Answer from the drawing. Dimensions are ordinates in mm from the lowest x, y and z of the part. A direction names the side the tool comes from. Give positions to 0.01 mm unless a question says otherwise; leave off trailing zeros. Order: outer loops, then holes, each group sorted by start corner. A loop starts at its lowest first (then second) coordinate and runs counter-clockwise, first axis right, second up.
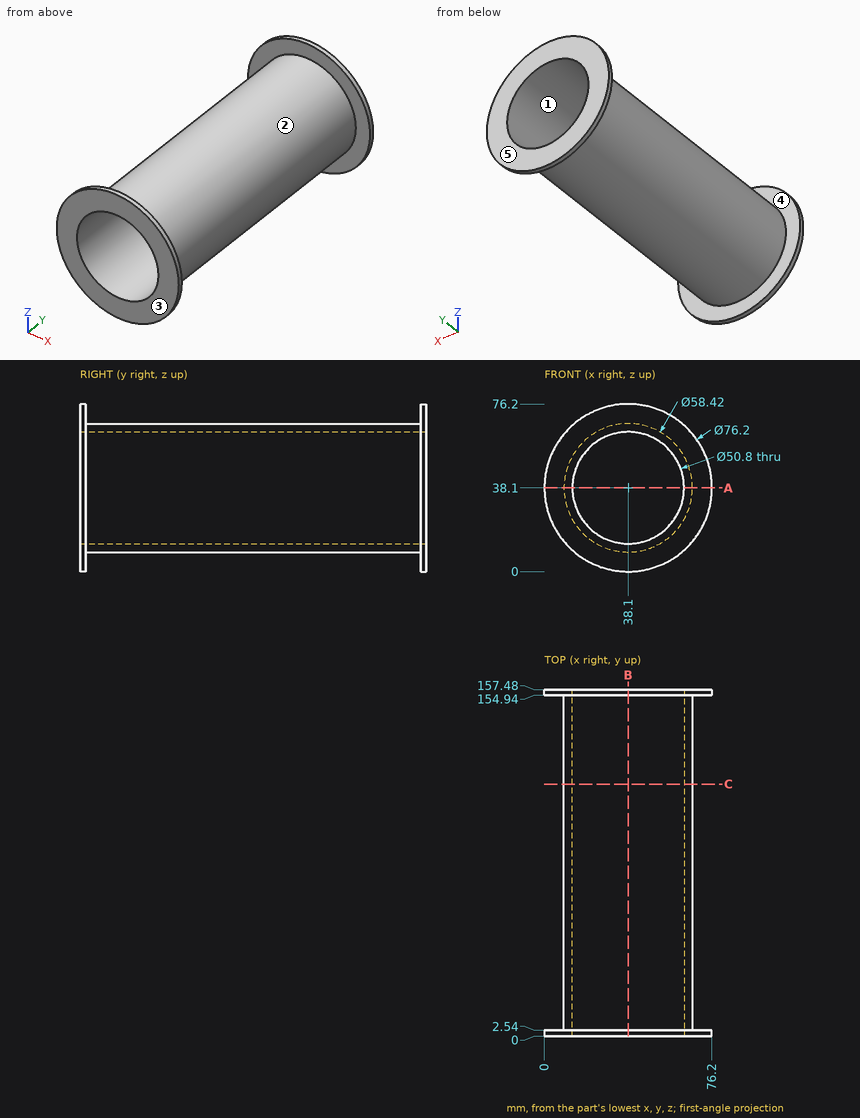
1. Which of the six approach directions +Z, -Z, +X, -X, +Y, -Y give full straight-line access (tool end or side, diameter ignored) to the marked faces 4 and 5?
Findings below:
face 4: none
face 5: +Z, -Z, +X, -X, +Y
2. The part is cut by section C-C (y = 114.5). Write down the section's boundary in (x, z).
Findings below:
outline: circle Ø58.42 at (38.1, 38.1); hole circle Ø50.8 at (38.1, 38.1)
3. The mould has two halves that part along Z. Classify the marked faces 1, 2 and 3: pulls with the +Z half, pulls with the -Z half, needs draft (parallel to the pull), parting line crosses it, or undercut.
Findings below:
face 1: undercut
face 2: parting line crosses it
face 3: needs draft
4. Given P1, Ø8, axis at y = 80.5, z = 66, coming from the +X side; P2, Ø1.5, axis at x = 21, y = 104.5, coming from the -Z side; P3, Ø6, axis at y = 120.5, z = 56, coming from the -X side; P4, Ø3, axis at x = 36.5, z = 16, coming from the -Y side, each flat-ended and moving along its own axis, determine where each tip first touches the part or whether it passes through.
Findings below:
P1: stops at x = 54.89
P2: stops at z = 13.89
P3: stops at x = 12.98
P4: passes through
5. Straight lines are drawn through the part: probe 1 along X at (y, z) = (89, 38); probe 2 along Y at (x, z) = (29.5, 5). For each, find the intervals that lie inside material, in ascending order.
Findings below:
probe 1: x = 8.89 to 12.7, 63.5 to 67.31
probe 2: y = 0 to 2.54, 154.94 to 157.48
6. The part is cut by section B-B (x = 38.1). Write down the section's boundary in (y, z), then the cut area to 3 significant figures.
Findings below:
outline: (0, 0) - (2.54, 0) - (2.54, 8.89) - (154.94, 8.89) - (154.94, 0) - (157.48, 0) - (157.48, 12.7) - (0, 12.7) - close; (0, 63.5) - (157.48, 63.5) - (157.48, 76.2) - (154.94, 76.2) - (154.94, 67.31) - (2.54, 67.31) - (2.54, 76.2) - (0, 76.2) - close
area: 1,290 mm2
7. The part is cut by section A-A (z = 38.1). Write down the section's boundary in (x, y), then the cut area to 3 significant figures.
Findings below:
outline: (0, 0) - (12.7, 0) - (12.7, 157.48) - (0, 157.48) - (0, 154.94) - (8.89, 154.94) - (8.89, 2.54) - (0, 2.54) - close; (63.5, 0) - (76.2, 0) - (76.2, 2.54) - (67.31, 2.54) - (67.31, 154.94) - (76.2, 154.94) - (76.2, 157.48) - (63.5, 157.48) - close
area: 1,290 mm2
